Check sheet for the modelled part. Datum: model origin and axes. Units: mm. Round coordinates to 2 decimals unless told otherwise and drop trailing zeros. Return JSON: item names as keys, results as strings.
from build123d import *

# Parameters (mm, degrees)
SKETCH3_R            = 27.94
BOSS_EXTRUDE2_DEPTH  = 122.46
SKETCH5_R            = 3.175
CUT_EXTRUDE1_DEPTH   = 129.676877488
SKETCH4_W            = 14
SKETCH4_H            = 6
SHELL1_START         = 3
SHELL1_OUTLINE_R     = 10.94
SHELL1_OUTLINE_R_2   = 6.175
SHELL1_DEPTH         = 116.46
SHELL1_2_OUTLINE_R   = 24.94
SHELL1_2_OUTLINE_R_2 = 10.94
SHELL1_2_DEPTH       = 10.72
SHELL1_START_2       = 109.72
SHELL1_3_OUTLINE_R   = 24.94
SHELL1_3_OUTLINE_R_2 = 10.94
SHELL1_3_DEPTH       = 9.74
SHELL1_START_3       = 25.72
SHELL1_4_OUTLINE_R   = 24.94
SHELL1_4_OUTLINE_R_2 = 10.94
SHELL1_4_DEPTH       = 9
SHELL1_START_4       = 46.72
SHELL1_5_OUTLINE_R   = 24.94
SHELL1_5_OUTLINE_R_2 = 10.94
SHELL1_5_DEPTH       = 9
SHELL1_START_5       = 67.72
SHELL1_6_OUTLINE_R   = 24.94
SHELL1_6_OUTLINE_R_2 = 10.94
SHELL1_6_DEPTH       = 9
SHELL1_START_6       = 88.72
SHELL1_7_OUTLINE_R   = 24.94
SHELL1_7_OUTLINE_R_2 = 10.94
SHELL1_7_DEPTH       = 9
BOSS_EXTRUDE3_START  = -119.46
BOSS_EXTRUDE3_DEPTH  = 116.46
SKETCH13_W           = 16.483162312
SKETCH13_H           = 6


# Read off the part's stored shape, not the designer's step: Shell1, Boss-Extrude3
with BuildPart() as part:
    # Sketch3 → Boss-Extrude2 (new body)
    with BuildSketch(Plane.XY):
        Circle(SKETCH3_R)
    extrude(amount=BOSS_EXTRUDE2_DEPTH)

    # Sketch5 → Cut-Extrude1 (cut, through all)
    with BuildSketch(Plane.XY.offset(122.46)):
        Circle(SKETCH5_R)
    extrude(amount=-CUT_EXTRUDE1_DEPTH, mode=Mode.SUBTRACT)

    # Sketch4 → Cut-Revolve1 (revolve, cut)
    with BuildSketch(Plane(origin=(0, 0, 0), x_dir=(1, 0, 0), z_dir=(0, 1, 0)), mode=Mode.PRIVATE) as cut_revolve1_sk:
        with Locations((-20.94, -103.72)):
            Rectangle(SKETCH4_W, SKETCH4_H)
        with Locations((-20.94, -82.72)):
            Rectangle(SKETCH4_W, SKETCH4_H)
        with Locations((-20.94, -61.72)):
            Rectangle(SKETCH4_W, SKETCH4_H)
        with Locations((-20.94, -40.72)):
            Rectangle(SKETCH4_W, SKETCH4_H)
        with Locations((-20.94, -19.72)):
            Rectangle(SKETCH4_W, SKETCH4_H)
    revolve(cut_revolve1_sk.sketch.rotate(Axis((0, 0, 122.46), (0, 0, -1)), 180), axis=Axis((0, 0, 122.46), (0, 0, -1)), mode=Mode.SUBTRACT)

    # Shell1 outline → Shell1 (cut)
    with BuildSketch(Plane.XY.offset(SHELL1_START)):
        Circle(SHELL1_OUTLINE_R)
        Circle(SHELL1_OUTLINE_R_2, mode=Mode.SUBTRACT)
    extrude(amount=SHELL1_DEPTH, mode=Mode.SUBTRACT)

    # Shell1 2 outline → Shell1 2 (cut)
    with BuildSketch(Plane.XY.offset(SHELL1_START)):
        Circle(SHELL1_2_OUTLINE_R)
        Circle(SHELL1_2_OUTLINE_R_2, mode=Mode.SUBTRACT)
    extrude(amount=SHELL1_2_DEPTH, mode=Mode.SUBTRACT)

    # Shell1 3 outline → Shell1 3 (cut)
    with BuildSketch(Plane.XY.offset(SHELL1_START_2)):
        Circle(SHELL1_3_OUTLINE_R)
        Circle(SHELL1_3_OUTLINE_R_2, mode=Mode.SUBTRACT)
    extrude(amount=SHELL1_3_DEPTH, mode=Mode.SUBTRACT)

    # Shell1 4 outline → Shell1 4 (cut)
    with BuildSketch(Plane.XY.offset(SHELL1_START_3)):
        Circle(SHELL1_4_OUTLINE_R)
        Circle(SHELL1_4_OUTLINE_R_2, mode=Mode.SUBTRACT)
    extrude(amount=SHELL1_4_DEPTH, mode=Mode.SUBTRACT)

    # Shell1 5 outline → Shell1 5 (cut)
    with BuildSketch(Plane.XY.offset(SHELL1_START_4)):
        Circle(SHELL1_5_OUTLINE_R)
        Circle(SHELL1_5_OUTLINE_R_2, mode=Mode.SUBTRACT)
    extrude(amount=SHELL1_5_DEPTH, mode=Mode.SUBTRACT)

    # Shell1 6 outline → Shell1 6 (cut)
    with BuildSketch(Plane.XY.offset(SHELL1_START_5)):
        Circle(SHELL1_6_OUTLINE_R)
        Circle(SHELL1_6_OUTLINE_R_2, mode=Mode.SUBTRACT)
    extrude(amount=SHELL1_6_DEPTH, mode=Mode.SUBTRACT)

    # Shell1 7 outline → Shell1 7 (cut)
    with BuildSketch(Plane.XY.offset(SHELL1_START_6)):
        Circle(SHELL1_7_OUTLINE_R)
        Circle(SHELL1_7_OUTLINE_R_2, mode=Mode.SUBTRACT)
    extrude(amount=SHELL1_7_DEPTH, mode=Mode.SUBTRACT)

    # Boss-Extrude3 outline → Boss-Extrude3 (add)
    with BuildSketch(Plane(origin=(0, 0, 0), x_dir=(-1, 0, 0), z_dir=(0, 0, -1)).offset(BOSS_EXTRUDE3_START)):
        with BuildLine():
            ThreePointArc((1, 27.922098775), (0, 27.94), (-1, 27.922098775))
            Line((-1, 27.922098775), (-1, 6.093490379))
            ThreePointArc((-1, 6.093490379), (0, 6.175), (1, 6.093490379))
            Line((1, 6.093490379), (1, 27.922098775))
        make_face()
        with BuildLine():
            Line((-27.922098775, -1), (-6.093490379, -1))
            ThreePointArc((-6.093490379, -1), (-6.175, 0), (-6.093490379, 1))
            Line((-6.093490379, 1), (-27.922098775, 1))
            ThreePointArc((-27.922098775, 1), (-27.94, 0), (-27.922098775, -1))
        make_face()
        with BuildLine():
            ThreePointArc((27.922098775, -1), (27.94, 0), (27.922098775, 1))
            Line((27.922098775, 1), (6.093490379, 1))
            ThreePointArc((6.093490379, 1), (6.175, 0), (6.093490379, -1))
            Line((6.093490379, -1), (27.922098775, -1))
        make_face()
        with BuildLine():
            Line((1, -27.922098775), (1, -6.093490379))
            ThreePointArc((1, -6.093490379), (0, -6.175), (-1, -6.093490379))
            Line((-1, -6.093490379), (-1, -27.922098775))
            ThreePointArc((-1, -27.922098775), (0, -27.94), (1, -27.922098775))
        make_face()
    extrude(amount=BOSS_EXTRUDE3_DEPTH)

    # Sketch13 → Cut-Revolve2 (revolve, cut)
    with BuildSketch(Plane(origin=(0, 0, 0), x_dir=(1, 0, 0), z_dir=(0, 1, 0)), mode=Mode.PRIVATE) as cut_revolve2_sk:
        with Locations((-22.145666886, -40.72)):
            Rectangle(SKETCH13_W, SKETCH13_H)
        with Locations((-22.145666886, -19.72)):
            Rectangle(SKETCH13_W, SKETCH13_H)
        with Locations((-22.145666886, -61.72)):
            Rectangle(SKETCH13_W, SKETCH13_H)
        with Locations((-22.145666886, -82.72)):
            Rectangle(SKETCH13_W, SKETCH13_H)
        with Locations((-22.145666886, -103.72)):
            Rectangle(SKETCH13_W, SKETCH13_H)
    revolve(cut_revolve2_sk.sketch.rotate(Axis((0, 0, 121.588746248), (0, 0, -1)), 180), axis=Axis((0, 0, 121.588746248), (0, 0, -1)), mode=Mode.SUBTRACT)


solid = part.part
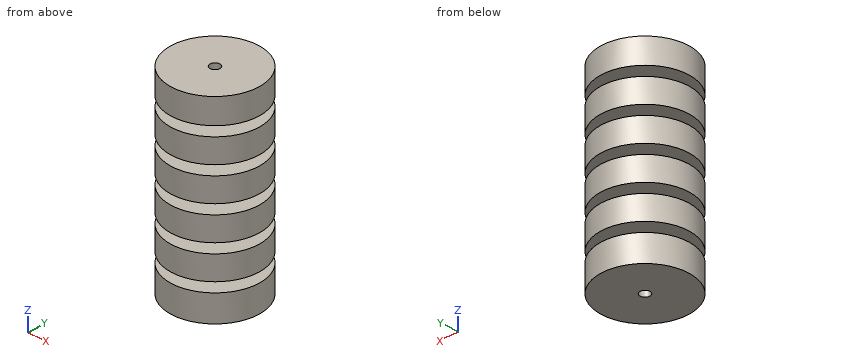
Q1. Go/stop test with flat-tipped pins: pin 1 (19 mm diameter, centred on x = -9.5, y = -7, fed in from -Z); pin 2 (3 mm diameter, centred on y = 17.5, z = 88, fed in from +X); pin 3 (12 mm diameter, centred on x = 8, z = 54.5, fed in from -Y); pin 4 (4 mm diameter, centred on x = 6.5, z = 41, fed in from -Y). Record where each tip stops, or that it passes through.
Results list:
{"pin 1": "z = 0", "pin 2": "x = 22.91", "pin 3": "y = -27.87", "pin 4": "y = -13.16"}
Q2. Section check A-A (z = 48.5). Count the separate pieces of the cut face and the enclosed holes in it, then the cut area to 3 significant figures.
Results list:
{"separate pieces": "1", "enclosed holes": "5", "area": "737 mm^2"}
Q3. Material ranges on line 1 (Z direction, x = -18.5, y = -0.5); line 2 (Y direction, x = 0, z = 72) (3 decimals); line 3 (Y direction, x = 0, z = 41.5) (3 decimals), recorded low to high.
Results list:
{"line 1": "0 to 16.72, 22.72 to 37.72, 43.72 to 58.72, 64.72 to 79.72, 85.72 to 100.72, 106.72 to 122.46", "line 2": "-27.94 to -3.175, 3.175 to 27.94", "line 3": "-13.904 to -3.175, 3.175 to 13.904"}
